Here's the drawing with two shaded views (mm, measured from the low corner). I have some questions. A direction names the side the tool comes from. Give positions to 0.01 mm unless a question says otherwise; leave off trailing zeros. Write each loop counter-clockwise with the first axis right and the second up, starting at its lowest first coordinate (ties: lowest second). Pieces come first, ordered by that corner, then holes. Notation, with made-up numbers: (-4, 62) - (7, 62) arc R22 ccw to (7, 74) - close; hole circle Ø9 at (-25, 8.25). An arc over 180 degrees is marked (long way). Use one line per item in the form item = value. Start each with the question number.
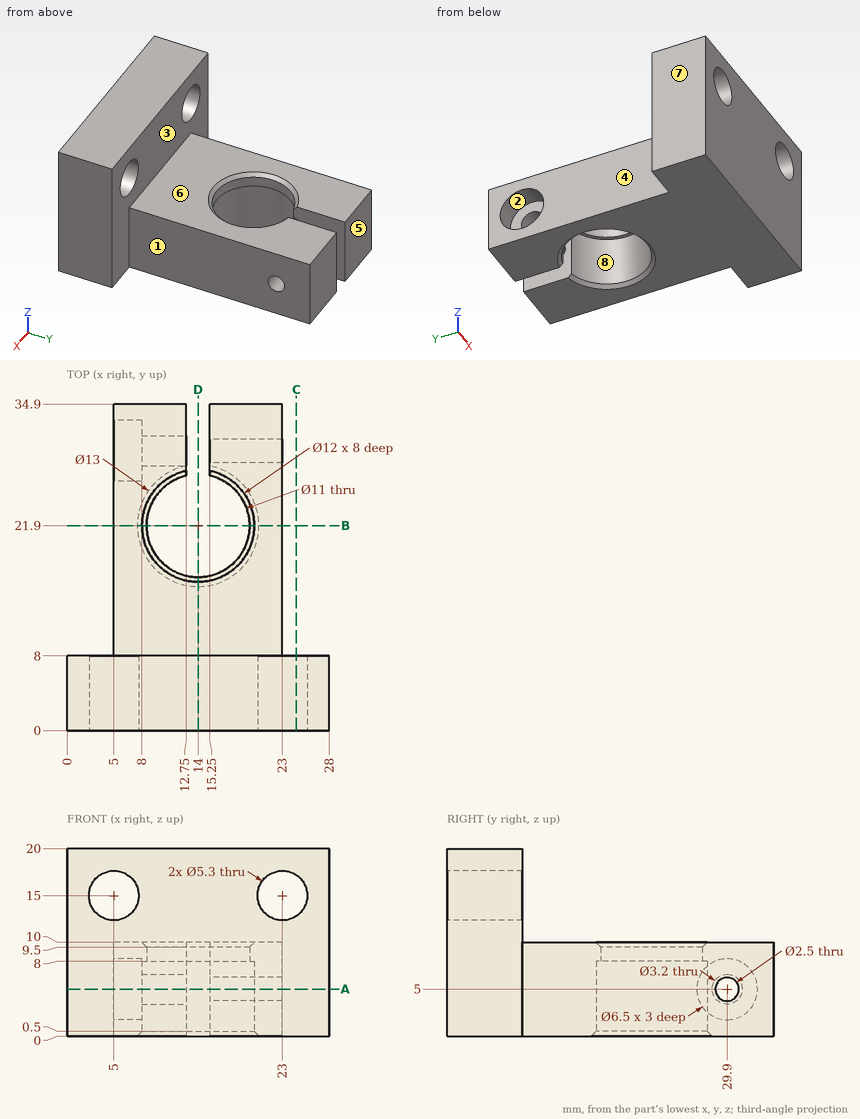
1. I want a section at D-D, the plane x = 14. List the corners of the cut face in (y, z) for me.
2. For P1, Ø6.5, axis at x = 14, y = 21.9, coming from the -Z side; P2, Ø5, axis at x = 9.5, y = 29.5, coming from the +Z side; P3, Ø8, axis at y = 18, z = 5.5, coming from the -X side; P4, Ø10.5, axis at y = 29.9, z = 5, coming from the +X side, each with a flat end and sliding along its axis, tell me the tip position at first contact or that it passes through.
3. Please list where these lines run through material, in increasing order: line 1 (X direction, y = 6, z = 15); line 2 (X direction, y = 29, z = 3.5); line 3 (Y direction, x = 6.2, z = 5).
4. I want a section at B-B, the plane y = 21.9. List the corners of the cut face in (x, z) for me, then the cut area to 3 significant figures.
5. We'd pull the mould along X, two halves only. Please class the marked faces 6, 7 and 8: pulls with the +X half, pulls with the -X half, needs draft (parallel to the pull), parting line crosses it, or undercut.
6. I want a section at A-A, the plane z = 5. List the corners of the cut face in (x, y) for me.
7. I want a section at C-C, the plane x = 24.5. List the corners of the cut face in (y, z) for me.
8. For the marked faces 1, 2, 3, 4 and 5, which set-ups out of +Z, -Z, +X, -X, +Y, -Y let a thin tool reach every point of the face, with its end or its side?
Result sheet:
q1.outline = (0, 0) - (15.4, 0) - (15.9, 0.5) - (15.9, 8) - (16.4, 8) - (16.4, 9.5) - (15.9, 10) - (8, 10) - (8, 20) - (0, 20) - close
q2.P1 = through
q2.P2 = 10
q2.P3 = 5
q2.P4 = 23
q3.line_1 = 0 to 2.35, 7.65 to 20.35, 25.65 to 28
q3.line_2 = 8 to 12.75, 15.25 to 23
q3.line_3 = 0 to 26.65, 33.15 to 34.9
q4.outline = (5, 0) - (7.5, 0) - (8, 0.5) - (8, 8) - (8.5, 8) - (8.5, 9.5) - (8, 10) - (5, 10) - close; (19.5, 8) - (20, 8) - (20, 0.5) - (20.5, 0) - (23, 0) - (23, 10) - (20, 10) - (19.5, 9.5) - close
q4.area = 61.5 mm2
q5.face_6 = needs draft
q5.face_7 = pulls with the -X half
q5.face_8 = undercut
q6.outline = (0, 0) - (28, 0) - (28, 8) - (23, 8) - (23, 28.65) - (15.25, 28.65) - (15.25, 27.77) arc R6 cw (long way) to (12.75, 27.77) - (12.75, 28.3) - (8, 28.3) - (8, 26.65) - (5, 26.65) - (5, 8) - (0, 8) - close; (5, 33.15) - (8, 33.15) - (8, 31.5) - (12.75, 31.5) - (12.75, 34.9) - (5, 34.9) - close; (15.25, 31.15) - (23, 31.15) - (23, 34.9) - (15.25, 34.9) - close
q7.outline = (0, 0) - (8, 0) - (8, 12.82) - (0, 12.82) - close; (0, 17.18) - (8, 17.18) - (8, 20) - (0, 20) - close
q8.face_1 = +Z, -Z, +X, +Y
q8.face_2 = -X
q8.face_3 = +Z, +Y
q8.face_4 = +Z, -Z, -X, +Y
q8.face_5 = +Z, -Z, +X, -X, +Y
